Work out the finished part from the listing and answer in its coordinate system (mm). Face numbers are marked on the shaded views. A direction names the side the tool comes from. Coordinates: 2 decimals unless noted, no trailing zeros. Loops run counter-clockwise (first coordinate to the right, second up) from the corner with the lowest first, then second, coordinate; pieces in that order, holes last.
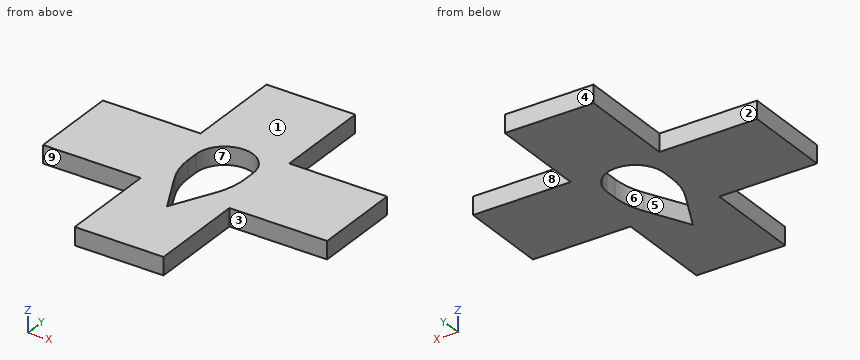
```python
from build123d import *

# Parameters (mm, degrees)
F1_DEPTH = 1.27


with BuildPart() as f1:
    # F0 (on Top) → F1 (new body)
    with BuildSketch(Plane.XY):
        Polygon((3.175, 10.16), (-3.175, 10.16), (-3.175, 3.175), (-10.16, 3.175), (-10.16, -3.175), (-3.175, -3.175), (-3.175, -10.16), (3.175, -10.16), (3.175, -3.175), (10.16, -3.175), (10.16, 3.175), (3.175, 3.175), align=None)
        with BuildLine():
            Line((-2.032, 0.183225), (-2.032, 1.016))
            ThreePointArc((-2.032, 1.016), (0, 3.048), (2.032, 1.016))
            Line((2.032, 1.016), (2.032, 0.183225))
            ThreePointArc((2.032, 0.183225), (1.896105, -0.98392), (1.49569, -2.08862))
            Line((1.49569, -2.08862), (0, -5.08))
            Line((0, -5.08), (-1.49569, -2.08862))
            ThreePointArc((-1.49569, -2.08862), (-1.896105, -0.98392), (-2.032, 0.183225))
        make_face(mode=Mode.SUBTRACT)
    extrude(amount=F1_DEPTH)


solid = f1.part
```
1. A cutting plane is placed at B-B, the plane y = -2.75. Give the vertices of the cut face in (x, z) (3 decimals), then the cut area to 3 significant figures.
2. For the marked faces 1, 2, 3, 4 and 5, determine the directions among +Z, -Z, +X, -X, +Y, -Y from which every point of the face is accessible in a straight line to the end or side of a thin tool.
3. Determine the mould class of the marked faces 6, 7, 8 and 9 for opening direction Y: released by +Y, released by -Y, zero draft, split by the parting line, or undercut.
4. Each of these flat-tipped pins is pushed along its axis until it touches: P1, Ø0.6, axis at y = 7, z = 1, coming from the +X side (3 decimals); P2, Ø0.6, axis at x = 8.5, z = 0.5, coming from the +Y side (3 decimals). Where does it stop, or does it pass through?
5. Straight lines are drawn through the part: probe 1 along X at (y, z) = (0.25, 0.25); probe 2 along Y at (x, z) = (3.5, 1.15) (3 decimals); probe 3 along X at (y, z) = (-2.25, 0.2) (3 decimals). For each, find the intervals that lie inside material, in ascending order.
6. A cutting plane is placed at A-A, the plane z = 0.9. Give the vertices of the cut face in (x, y) (3 decimals), then the cut area to 3 significant figures.
7. A cutting plane is placed at D-D, the plane y = -0.25. Give the vertices of the cut face in (x, z).
8. A cutting plane is placed at C-C, the plane x = 5. Give the vertices of the cut face in (y, z) (3 decimals).
Answers below:
1. outline: (-10.16, 0) - (-1.165, 0) - (-1.165, 1.27) - (-10.16, 1.27) - close; (1.165, 0) - (10.16, 0) - (10.16, 1.27) - (1.165, 1.27) - close
1. area: 22.8 mm2
2. face 1: +Z, +X, -X, +Y, -Y
2. face 2: +Z, -Z, -X, +Y
2. face 3: +Z, -Z, +X, -Y
2. face 4: +Z, -Z, +X, -X, +Y
2. face 5: +Z, -Z
3. face 6: undercut
3. face 7: undercut
3. face 8: released by +Y
3. face 9: released by -Y
4. P1: stops at x = 3.175
4. P2: stops at y = 3.175
5. probe 1: x = -10.16 to -2.03, 2.03 to 10.16
5. probe 2: y = -3.175 to 3.175
5. probe 3: x = -10.16 to -1.415, 1.415 to 10.16
6. outline: (-10.16, -3.175) - (-3.175, -3.175) - (-3.175, -10.16) - (3.175, -10.16) - (3.175, -3.175) - (10.16, -3.175) - (10.16, 3.175) - (3.175, 3.175) - (3.175, 10.16) - (-3.175, 10.16) - (-3.175, 3.175) - (-10.16, 3.175) - close; hole (-2.032, 0.183) arc R5.08 ccw to (-1.496, -2.089) - (0, -5.08) - (1.496, -2.089) arc R5.08 ccw to (2.032, 0.183) - (2.032, 1.016) arc R2.032 ccw to (-2.032, 1.016) - close
6. area: 195 mm2
7. outline: (-10.16, 0) - (-2.01, 0) - (-2.01, 1.27) - (-10.16, 1.27) - close; (2.01, 0) - (10.16, 0) - (10.16, 1.27) - (2.01, 1.27) - close
8. outline: (-3.175, 0) - (3.175, 0) - (3.175, 1.27) - (-3.175, 1.27) - close
